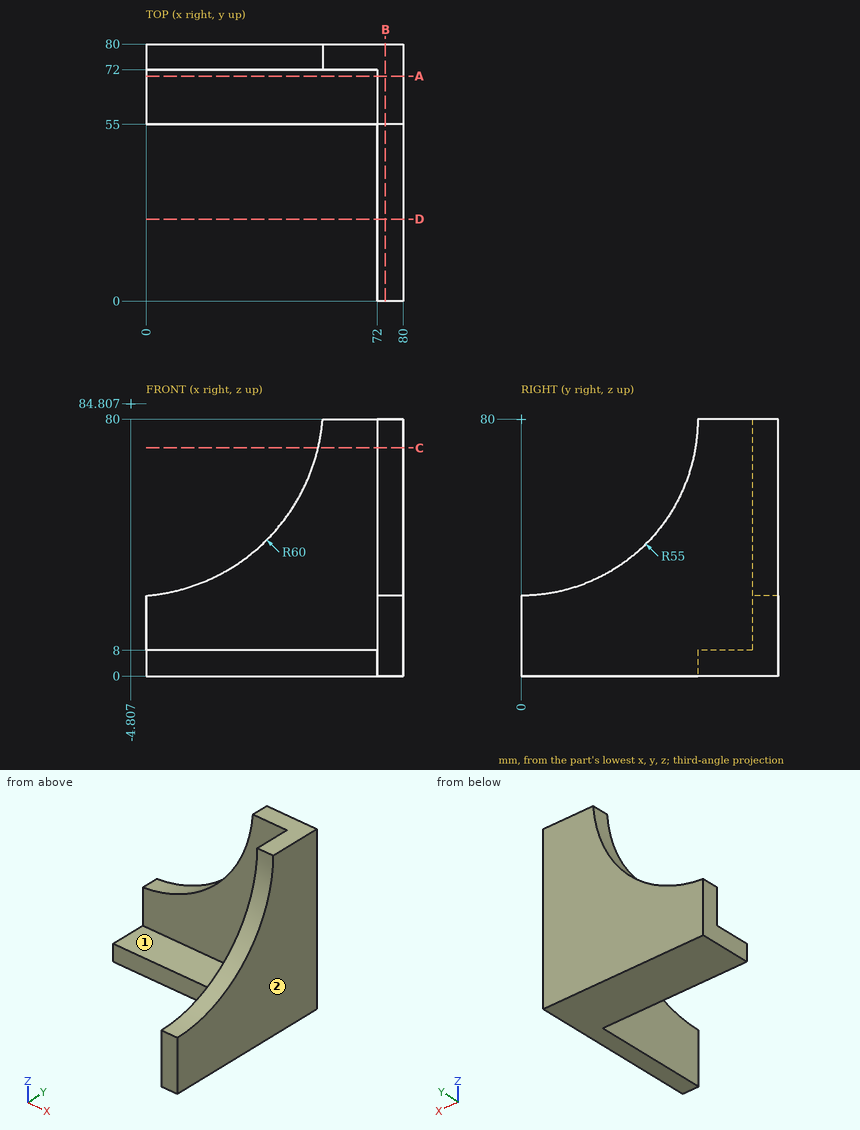
Geometry check sheet. Reference: drawing and pictorial views, mm from the part's lowest x, y, z. A direction names the side the tool comes from. Round coordinates to 2 decimals unless told otherwise and drop trailing zeros. Write each loop counter-clockwise with the first axis right and the second up, starting at its lowest first coordinate (ties: lowest second). Pieces come first, ordered by that corner, then holes. Notation, with made-up numbers: (-3.75, 46.5) -> (4.25, 46.5) arc R20 cw to (4.25, 64.5) -> close; hole circle Ø2 at (49.25, 85.5). An arc over 180 degrees is marked (long way). Put each result on its own line as item: value.
1) Cross-section at D-D, the plane y = 25.5. Enter the section's corners in (x, z), plus the area to 3 significant figures.
Recorded:
outline: (72, 0) -> (80, 0) -> (80, 31.27) -> (72, 31.27) -> close
area: 250 mm2
2) Cross-section at B-B, the plane x = 74.5. Enter the section's corners in (y, z).
Recorded:
outline: (0, 0) -> (80, 0) -> (80, 80) -> (55, 80) arc R55 cw to (0, 25) -> close
3) Depth check by flat-ended pin: P1, Ø10, axis at x = 31, y = 70.5, coming from the -Z side; P2, Ø5, axis at y = 39.5, z = 11.5, coming from the -X side; P3, Ø9, axis at x = 49.5, z = 5, coming from the -Y side; P4, Ø6, axis at x = 71, z = 59.5, coming from the -Y side. Enter the tip coordinate at first touch or a pass-through.
Recorded:
P1: stops at z = 0
P2: stops at x = 72
P3: stops at y = 55
P4: stops at y = 49.81
4) Access from +Z, -Z, +X, -X, +Y, -Y to the whole of each face (thin tool, end or side, straight path). Record for the marked faces 1 and 2.
Recorded:
face 1: +Z, -X, -Y
face 2: +Z, -Z, +X, +Y, -Y
5) Cross-section at C-C, the plane z = 71. Enter the section's corners in (x, y).
Recorded:
outline: (53.58, 72) -> (72, 72) -> (72, 54.26) -> (80, 54.26) -> (80, 80) -> (53.58, 80) -> close
6) Cross-section at A-A, the plane y = 70. Enter the section's corners in (x, z), plus the area to 3 significant figures.
Recorded:
outline: (0, 0) -> (80, 0) -> (80, 80) -> (72, 80) -> (72, 8) -> (0, 8) -> close
area: 1,220 mm2
7) Thickness scan on probe 1 along Y at (x, z) = (18, 6); probe 2 along Y at (x, z) = (55, 50.5); probe 3 along Z at (x, y) = (25, 56.5). Record the ranges inside material, lowest first. Write a range as from..to.
Recorded:
probe 1: y = 55..80
probe 2: y = 72..80
probe 3: z = 0..8
